from build123d import *

# Parameters (mm, degrees)
F0_R     = 15.3
F1_DEPTH = 96
F3_D     = 17.95
F3_DEPTH = 65
F3_TIP   = 5.3927240558
F4_SIZE2 = 10
F4_SIZE  = 5
F6_D     = 4
F6_DEPTH = 1
F6_START = 66.2017213
F6_TIP   = 1.2017212381
F8_D     = 17.95
F8_DEPTH = 5
F8_TIP   = 5.3927240558


with BuildPart() as f1:
    # F0 (on Top) → F1 (new body)
    with BuildSketch(Plane.XY):
        Circle(F0_R)
    extrude(amount=F1_DEPTH)

    # F3
    with Locations(Plane.XY.offset(96)):
        with Locations((0, 0)):
            Hole(F3_D / 2, depth=F3_DEPTH)
            with Locations((0, 0, -(F3_DEPTH + F3_TIP / 2))):  # 118° drill point
                Cone(0, F3_D / 2, F3_TIP, mode=Mode.SUBTRACT)

    # F4
    f4_edges = [f1.edges().sort_by_distance(p)[0] for p in [
        (-15.3, 0, 96),
    ]]
    f4_side = f1.faces().sort_by_distance((-14.867251, 0, 96))[0]
    chamfer(f4_edges, length=F4_SIZE, length2=F4_SIZE2, reference=f4_side)

    # F6
    # its depths count from where the whole tool has entered the part; down to there all is cleared
    with Locations(Plane.XY.offset(96)):
        with Locations((0, 8.975)):
            Hole(F6_D / 2, depth=F6_START)
    with Locations(Plane.XY.offset(96).offset(-F6_START)):
        with Locations((0, 8.975)):
            Hole(F6_D / 2, depth=F6_DEPTH)
            with Locations((0, 0, -(F6_DEPTH + F6_TIP / 2))):  # 118° drill point
                Cone(0, F6_D / 2, F6_TIP, mode=Mode.SUBTRACT)

    # F8
    with Locations(Plane(origin=(0, 0, 0), x_dir=(1, 0, 0), z_dir=(0, 0, -1))):
        with Locations((0, 0)):
            Hole(F8_D / 2, depth=F8_DEPTH)
            with Locations((0, 0, -(F8_DEPTH + F8_TIP / 2))):  # 118° drill point
                Cone(0, F8_D / 2, F8_TIP, mode=Mode.SUBTRACT)


solid = f1.part
Design review of the part built by this model. Coordinates are the model's own, in mm. A direction names the side the tool comes from. Give positions to 0.01 mm unless a question says otherwise; leave off trailing zeros. Loops run counter-clockwise (first coordinate to the right, second up) from the corner with the lowest first, then second, coordinate; pieces in that order, holes last. Notation, with made-up numbers: (63.5, 51.5) - (115.5, 51.5) arc R16 cw to (115.5, 57.5) - close; hole circle Ø8 at (18.25, 50). An arc over 180 degrees is marked (long way). Use CSV: the item, a comma, the result in double quotes. Start each with the question number.
1. Insertion check: P1, Ø2.5, axis at x = 0, y = 8.975, coming from the +Z side; P2, Ø16, axis at x = 0, y = 0, coming from the +Z side; P3, Ø1.5, axis at y = 7, z = 27, coming from the -X side. Each pin has a flat end and moves straight along its axis. Give the tip position at first contact, or say it passes through.
2. Wall thickness on L1, parallel to Y at x = 0, z = 65 (3 decimals); L2, parallel to Y at x = 0, z = 1.85 (3 decimals); L3, parallel to X at y = 8, z = 84.5: over which ranges is each line inside the solid? List them lowest first.
3. Add section B-B (z = 34). State the section outline as (x, y) points (3 decimals).
4. Machinability: for faces 5 (the flat face through (-0.8, -9.1, 96)), 6 (the cylindrical face through (0.367, -8.968, 63.045)), which of the approach directions +Z, -Z, +X, -X, +Y, -Y give a long, thin tool a straight path to every point of the face, cutting with its end or side? Answer none if there is none.
5. Draft analysis for pull direction X (two halves, no side actions). For faces 1 (the conical face through (10.123, 3.188, 95.374)), 2 (the conical face through (-0.338, -1.522, 26.544)), 3 (the cylindrical face through (-8.56, -2.7, 2.54)), 4 (the flat face through (7, -7, 0)), state which applies: released by +X, released by -X, zero draft, split by the parting line, or undercut.
6. Add section A-A (z = 8). State the section outline as (x, y) points, plus the area to 3 significant figures.
Results found:
1,P1,"stops at z = 28.35"
1,P2,"stops at z = 30.41"
1,P3,"stops at x = -13.97"
2,L1,"y = -15.3 to -8.975, 10.975 to 15.3"
2,L2,"y = -15.3 to -8.975, 8.975 to 15.3"
2,L3,"x = -13.04 to -4.07, 4.07 to 13.04"
3,outline,"circle Ø30.6 at (0, 0); hole (-1.988, 8.752) arc R8.975 ccw (long way) to (1.988, 8.752) arc R2 ccw (long way) to start"
4,face 5,"+Z, +X, -X, +Y, -Y"
4,face 6,"+Z"
5,face 1,"split by the parting line"
5,face 2,"undercut"
5,face 3,"undercut"
5,face 4,"zero draft"
6,outline,"circle Ø30.6 at (0, 0); hole circle Ø7.96 at (0, 0)"
6,area,"686 mm²"
